Read the model definition and answer for the solid it produces. Units are mm, in the model's axes. Coordinates: 2 decimals unless noted, no trailing zeros. Write each loop counter-clockwise with the first axis right and the second up, starting at its lowest first coordinate (ties: lowest second). Pieces come first, ordered by that corner, then holes. Notation, with made-up numbers: (77.25, 63) -> (105.25, 63) arc R14 ccw to (105.25, 83) -> close; hole circle Ø1 at (-18.75, 62). An arc over 180 degrees is marked (long way). Write item = value, one per line. Start each with the question number.
1) Section A-A (z = 25.5) is taken. Determine the outline of the cut face in (x, y).
2) Find the intervals of material crossed by line 1 along Z through (x, y) = (3.1, -156.5); line 2 along Z through (x, y) = (1.3, -145); line 3 along Y through (x, z) = (2.25, 12.5), in increasing order. Write a range as from..to.
3) Section C-C (y = -143) is taken. Determine the outline of the cut face in (x, z), plus the area to 3 significant figures.
4) Section B-B (x = 3.15) is taken. Determine the outline of the cut face in (y, z).
5) A flat-ended cylindrical pin translates along its axis: pin 1 Ø2.5 at (x, y) = (2.5, -170) entering from +Z. Find the tip coordinate at first contact, or state that the pin passes through.
6) Section D-D (y = 79) is taken. Determine the outline of the cut face in (x, z), plus the area to 3 significant figures.
from build123d import *

# Parameters (mm, degrees)
F1_DEPTH = 5.08
F2_R     = 12.7
F3_DEPTH = 12.7


with BuildPart() as f1:
    # F0 (on Right) → F1 (new body)
    with BuildSketch(Plane.YZ):
        Polygon((143.104023, 0), (143.104023, 13.61572), (-132.544885, 78.375299), (-132.544885, 37.545515), (-187.095977, 37.545515), (-187.095977, 0), (-132.544885, 0), align=None)
    extrude(amount=F1_DEPTH)

    # F2 (on face) → F3 (cut)
    with BuildSketch(Plane.YZ.offset(5.08)):
        with Locations((-160.357416, 17.813968)):
            Circle(F2_R)
    extrude(amount=-F3_DEPTH, mode=Mode.SUBTRACT)


solid = f1.part
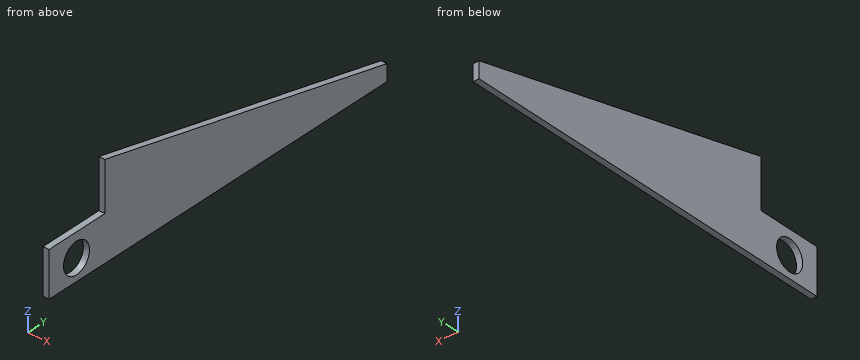
Answer key:
q1.outline = (0, -187.1) -> (5.08, -187.1) -> (5.08, -170.47) -> (0, -170.47) -> close; (0, -150.25) -> (5.08, -150.25) -> (5.08, 92.52) -> (0, 92.52) -> close
q2.line_1 = 0..5.71, 29.91..37.55
q2.line_2 = 0..37.55
q2.line_3 = -187.1..-171.89, -148.82..143.1
q3.outline = (0, 0) -> (5.08, 0) -> (5.08, 37.55) -> (0, 37.55) -> close
q3.area = 191 mm^2
q4.outline = (-187.1, 0) -> (143.1, 0) -> (143.1, 13.62) -> (-132.54, 78.38) -> (-132.54, 37.55) -> (-187.1, 37.55) -> close; hole circle Ø25.4 at (-160.36, 17.81)
q5.pin_1 = 37.55
q6.outline = (0, 0) -> (5.08, 0) -> (5.08, 28.68) -> (0, 28.68) -> close
q6.area = 146 mm^2
